Design review of the part shown in the three views and the two pictorial views. Dimensions are in mm from the part's minimum x, y and z. A direction names the side the tool comes from. Round coordinates to 2 decimals unless told otherwise and drop trailing zeros. Loops run counter-clockwise (first coordinate to the right, second up) from the corner with the lowest first, then second, coordinate; pieces in that order, holes last. Notation, with made-up numbers: (69, 63) -> (82, 63) arc R7 cw to (82, 75) -> close; hole circle Ø4 at (56.25, 88). An arc over 180 degrees is marked (long way). Use a Markdown table: item, result. Add a question column.
1) Insertion check: pin 1 (4 mm diameter, centred on x = 13, z = 60, fed in from -Y); pin 2 (1.9 mm diameter, centred on x = 27, z = 60, fed in from -Y); pin 3 (2 mm diameter, centred on x = 22.5, z = 77.5, fed in from +Y). Each pin has a flat end and moves straight along its axis. Give the tip position at first contact, or say it passes through.
2) Consider section B-B on x = 20. Give the boundary of the cut face in (y, z).
3) For the marked faces 1 and 2, list the 3-axis set-ups (+Z, -Z, +X, -X, +Y, -Y) from which the entire face can be reached by the end or side of a thin tool; tool diameter is ignored.
4) Consider section A-A on y = 23. Give the boundary of the cut face in (x, z), plus the area to 4 significant figures.
5) Wall thickness on probe 1 along X at (y, z) = (1, 15); probe 2 along Z at (x, y) = (13, 1); probe 3 along Z at (x, y) = (38.5, 38): over which ranges is each line inside the solid? List them lowest first.
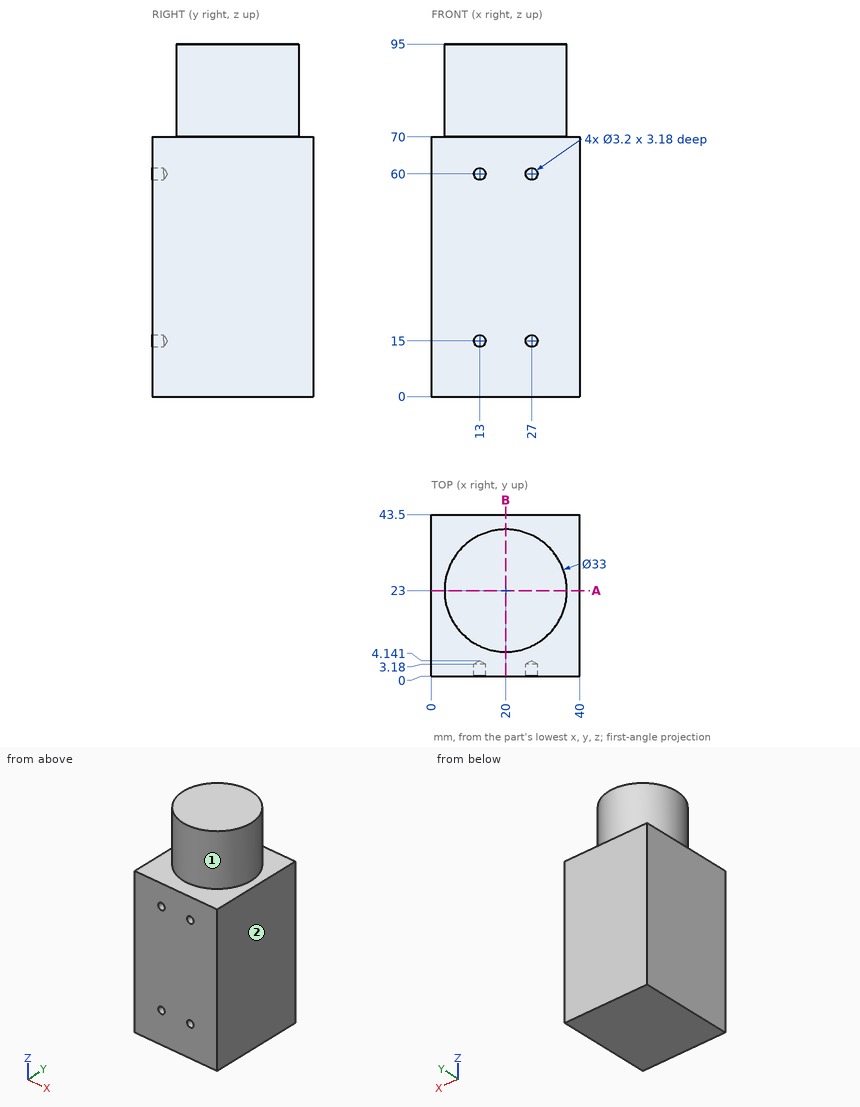
Result set:
| question | item | result |
|---|---|---|
| 1 | pin 1 | y = 0 |
| 1 | pin 2 | y = 3.57 |
| 1 | pin 3 | y = 39.43 |
| 2 | outline | (0, 0) -> (43.5, 0) -> (43.5, 70) -> (39.5, 70) -> (39.5, 95) -> (6.5, 95) -> (6.5, 70) -> (0, 70) -> close |
| 3 | face 1 | +Z |
| 3 | face 2 | +Z, -Z, +X, +Y, -Y |
| 4 | outline | (0, 0) -> (40, 0) -> (40, 70) -> (36.5, 70) -> (36.5, 95) -> (3.5, 95) -> (3.5, 70) -> (0, 70) -> close |
| 4 | area | 3,625 mm2 |
| 5 | probe 1 | 0 to 11.4, 14.6 to 25.4, 28.6 to 40 |
| 5 | probe 2 | 0 to 13.4, 16.6 to 58.4, 61.6 to 70 |
| 5 | probe 3 | 0 to 70 |
